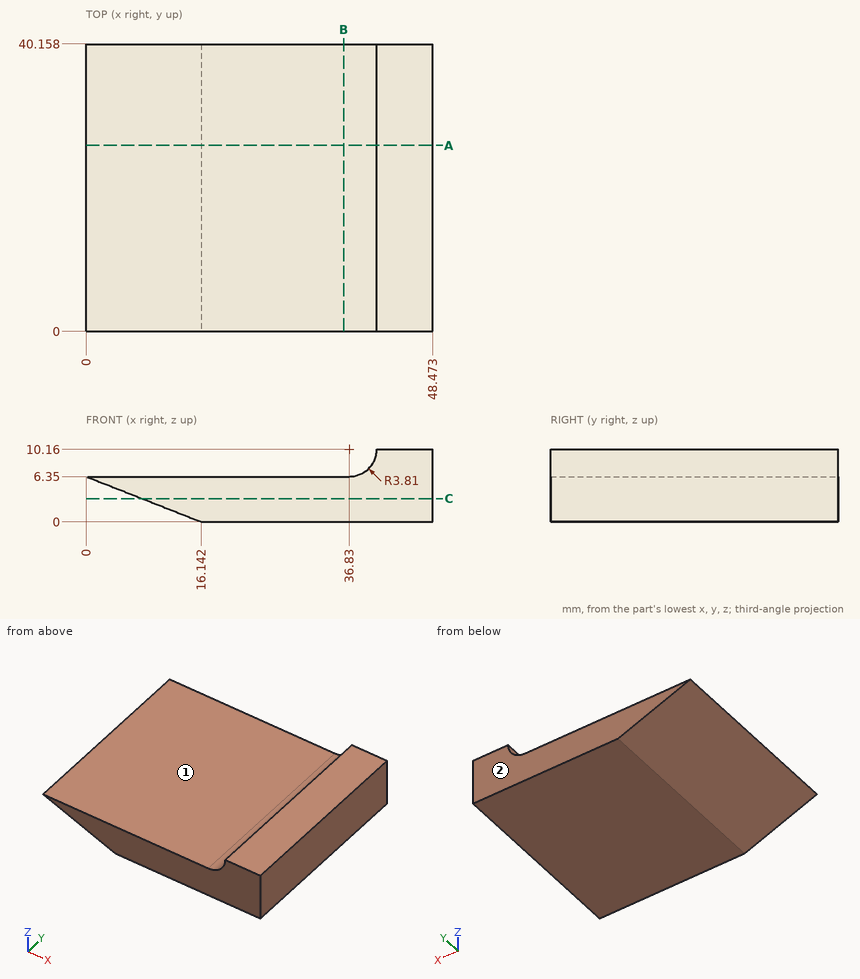
Could you check a few things on this drawing? It's one solid part, dimensions in mm from its lowest x, y, z. A direction names the side the tool comes from. Round coordinates to 2 decimals unless told otherwise and drop trailing zeros. Order: outer loops, then holes, each group sorted by start corner. A loop starts at its lowest first (then second) coordinate and runs counter-clockwise, first axis right, second up. Notation, with made-up numbers: M 20.25,79.25 L 46.25,79.25 A13 cw 46.25,99.25 Z; hole C 72.5,-4 d6. An arc over 180 degrees is marked long. Use a Markdown table: item, result.
1) Imagine slicing it at A-A (y = 26). List the corners of the cut face in (x, z) for me.
Geometry says:
| item | result |
|---|---|
| outline | M 0,6.35 L 16.14,0 L 48.47,0 L 48.47,10.16 L 40.64,10.16 A3.81 cw 36.83,6.35 Z |
2) Imagine slicing it at C-C (z = 3.25). List the corners of the cut face in (x, y) for me, then the cut area to 3 significant figures.
Geometry says:
| item | result |
|---|---|
| outline | M 7.88,0 L 48.47,0 L 48.47,40.16 L 7.88,40.16 Z |
| area | 1,630 mm² |
3) I'm going to push flat-ended pins straight in: P1, Ø5, axis at x = 17.5, y = 24.5, coming from the +Z side; P2, Ø3, axis at x = 5, y = 13, coming from the -Z side; P3, Ø4, axis at x = 19.5, y = 35.5, coming from the -Z side. Where does each tip first touch, or does it pass through?
Geometry says:
| item | result |
|---|---|
| P1 | stops at z = 6.35 |
| P2 | stops at z = 3.79 |
| P3 | stops at z = 0 |
4) Imagine slicing it at B-B (x = 36). List the corners of the cut face in (y, z) for me, then the cut area to 3 significant figures.
Geometry says:
| item | result |
|---|---|
| outline | M 0,0 L 40.16,0 L 40.16,6.35 L 0,6.35 Z |
| area | 255 mm² |
5) If I drill on line 1 along Z through (x, y) = (23, 14); line 2 along X through (y, z) = (17, 7.5) (1 decimal); line 3 along X through (y, z) = (20, 6.75) (1 decimal), over which ranges is the centre line in solid material (lowest first)?
Geometry says:
| item | result |
|---|---|
| line 1 | z = 0 to 6.35 |
| line 2 | x = 39.6 to 48.5 |
| line 3 | x = 38.5 to 48.5 |
6) On a 3-axis mill with a long thin cutter (end or side, diameter ignored), from which of +Z, -Z, +X, -X, +Y, -Y can I reach the whole of each face in a straight line? I mean the marked faces 1 and 2. Say none if no direction works.
Geometry says:
| item | result |
|---|---|
| face 1 | +Z, -X, +Y, -Y |
| face 2 | +Z, -Z, +X, -X, +Y |
